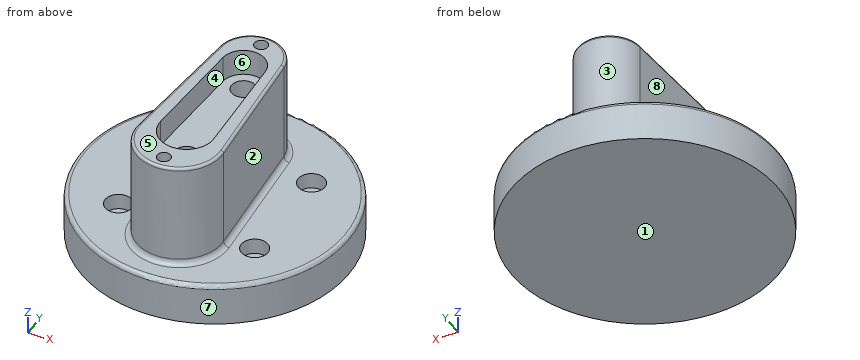
```python
from build123d import *

# Parameters (mm, degrees)
SKETCH_R        = 25
PAD_DEPTH       = 8
PAD001_DEPTH    = 20
SKETCH002_R     = 2.5
POCKET_DEPTH    = 3
POCKET001_DEPTH = 5
SKETCH004_R     = 2.25
POCKET002_DEPTH = 5
SKETCH005_R     = 1.25
POCKET003_DEPTH = 5
FILLET_R        = 0.75
FILLET001_R     = 1
FILLET002_R     = 0.5


with BuildPart() as part:
    # Sketch → Pad (new body)
    with BuildSketch(Plane.XY):
        Circle(SKETCH_R)
    extrude(amount=PAD_DEPTH)

    # Sketch001 (on Face3 of Pad) → Pad001 (join)
    with BuildSketch(Plane.XY.offset(8)):
        with BuildLine():
            ThreePointArc((5.980892, 13.018408), (0, 18.539936), (-5.980892, 13.018408))
            Line((-5.980892, 13.018408), (-7.974522, -11.901974))
            ThreePointArc((-7.974522, -11.901974), (0, -20.539936), (7.974522, -11.901974))
            Line((7.974522, -11.901974), (5.980892, 13.018408))
        make_face()
    extrude(amount=PAD001_DEPTH)

    # Sketch002 (on Face3 of Pad001) → Pocket (cut)
    with BuildSketch(Plane.XY.offset(8)):
        with Locations((12.79, 10)):
            Circle(SKETCH002_R)
        with Locations((12.79, -10)):
            Circle(SKETCH002_R)
        with Locations((-12.79, -10)):
            Circle(SKETCH002_R)
        with Locations((-12.79, 10)):
            Circle(SKETCH002_R)
    extrude(amount=-POCKET_DEPTH, mode=Mode.SUBTRACT)

    # Sketch003 (on Face14 of Pocket) → Pocket001 (cut)
    with BuildSketch(Plane.XY.offset(28)):
        with BuildLine():
            ThreePointArc((3.995019, 10.222031), (0, 14.02248), (-3.995019, 10.222031))
            Line((-3.995019, 10.222031), (-4.993774, -9.77304))
            ThreePointArc((-4.993774, -9.77304), (0, -15.02248), (4.993774, -9.77304))
            Line((4.993774, -9.77304), (3.995019, 10.222031))
        make_face()
    extrude(amount=-POCKET001_DEPTH, mode=Mode.SUBTRACT)

    # Sketch004 (on Face21 of Pocket001) → Pocket002 (cut)
    with BuildSketch(Plane.XY.offset(23)):
        with Locations((0, 10.025)):
            Circle(SKETCH004_R)
        with Locations((0, -10.025)):
            Circle(SKETCH004_R)
    extrude(amount=-POCKET002_DEPTH, mode=Mode.SUBTRACT)

    # Sketch005 (on Face14 of Pocket002) → Pocket003 (cut)
    with BuildSketch(Plane.XY.offset(28)):
        with Locations((0, 16.24)):
            Circle(SKETCH005_R)
        with Locations((0, -18)):
            Circle(SKETCH005_R)
    extrude(amount=-POCKET003_DEPTH, mode=Mode.SUBTRACT)

    # Fillet
    fillet_edges = [part.edges().sort_by_distance(p)[0] for p in [
        (-25, 0, 8),
    ]]
    fillet(fillet_edges, radius=FILLET_R)

    # Fillet001
    fillet001_edges = [part.edges().sort_by_distance(p)[0] for p in [
        (0, -20.539936, 8),
    ]]
    fillet(fillet001_edges, radius=FILLET001_R)

    # Fillet002
    fillet002_edges = [part.edges().sort_by_distance(p)[0] for p in [
        (6.977707, 0.558217, 28),
    ]]
    fillet(fillet002_edges, radius=FILLET002_R)


solid = part.part
```
Here's how the part is built. I have some questions about the finished solid (model axes, mm). Face numbers are marked on the shaded views. A direction names the side the tool comes from. Coordinates: 2 decimals unless noted, no trailing zeros. Order: outer loops, then holes, each group sorted by start corner. A loop starts at its lowest first (then second) coordinate and runs counter-clockwise, first axis right, second up.
Item 1: I'm going to push flat-ended pins straight in: pin 1 Ø0.8 at (x, y) = (0, 16.5) entering from +Z; pin 2 Ø3 at (y, z) = (-2, 22.5) entering from -X; pin 3 Ø4 at (x, y) = (19, 0.5) entering from -Z; pin 4 Ø8 at (x, y) = (13, -15) entering from +Z. Where does each tip first touch, or does it pass through?
Response values:
pin 1: stops at z = 23
pin 2: stops at x = -7.3
pin 3: stops at z = 0
pin 4: stops at z = 8
Item 2: I need wall thicknesses on probe 1 along Y at (x, z) = (0, 22.05) (3 decimals); probe 2 along Y at (x, z) = (0, 25.15); probe 3 along Z at (x, y) = (-8, 2). Which ranges of each line are inside material? Lowest first, please.
Response values:
probe 1: y = -20.54 to -12.275, -7.775 to 7.775, 12.275 to 18.54
probe 2: y = -20.54 to -19.25, -16.75 to -15.02, 14.02 to 14.99, 17.49 to 18.54
probe 3: z = 0 to 8
Item 3: Which directions (+Z, -Z, +X, -X, +Y, -Y) give clear straight access to the entire face, cutting with the end or side of a thin tool? Please do the marked faces 1, 2, 3 and 4.
Response values:
face 1: -Z, +X, -X, +Y, -Y
face 2: +Z, +X, +Y
face 3: +Z, +Y
face 4: +Z
Item 4: If we section it at C-C, the plane z = 20.25: List the corners of the cut face in (x, y) for me (3 decimals).
Response values:
outline: (-7.975, -11.902) arc R8 ccw (long way) to (7.975, -11.902) - (5.981, 13.018) arc R6 ccw to (-5.981, 13.018) - close; hole circle Ø4.5 at (0, -10.025); hole circle Ø4.5 at (0, 10.025)
Item 5: If we section it at B-B, the plane z = 15.75: List the corners of the cut face in (x, y) for me, then the cut area to 3 significant figures.
Response values:
outline: (-7.97, -11.9) arc R8 ccw (long way) to (7.97, -11.9) - (5.98, 13.02) arc R6 ccw to (-5.98, 13.02) - close
area: 509 mm2
Item 6: Thinking about a two-plate mould opening in Y: for the marked faces 5, 6, 7 and 8, which applies, pulls with the +Y half, pulls with the -Y half, needs draft (parallel to the pull), parting line crosses it, or undercut?
Response values:
face 5: needs draft
face 6: undercut
face 7: parting line crosses it
face 8: pulls with the +Y half
